Read the model definition and answer for the solid it produces. Units are mm, in the model's axes. Face numbers are marked on the shaded views. A direction names the side the tool comes from. Give positions to 0.01 mm unless a question says otherwise; leave off trailing zeros. Loops run counter-clockwise (first coordinate to the right, second up) from the corner with the lowest first, then second, coordinate; pieces in that order, holes last. Notation, with made-up numbers: (43, 37.25) - (47, 37.25) arc R17 cw to (47, 42.25) - close; hole circle Ø6 at (-11, 55.25). An arc over 180 degrees is marked (long way). Write item = value, one per line.
```python
from build123d import *

# Parameters (mm, degrees)
ESBO_O1_W                = 8.5
ESBO_O1_H                = 8.5
ESBO_O1_W_2              = 3.29
ESBO_O1_H_2              = 3.29
RESSALTO_EXTRUS_O1_DEPTH = 7.3
ESBO_O2_W                = 40
ESBO_O2_H                = 40
RESSALTO_EXTRUS_O2_DEPTH = 10
FILETE1_R                = 10
FILETE2_R                = 10
FILETE3_R                = 5
ESBO_O3_W                = 0.5
ESBO_O3_H                = 1.5
ESBO_O3_W_2              = 1.5
ESBO_O3_H_2              = 0.5
CORTE_EXTRUS_O1_DEPTH    = 5
FILETE4_R                = 1


with BuildPart() as part:
    # Esboço1 → Ressalto-extrusão1 (new body)
    with BuildSketch(Plane.XY):
        Rectangle(ESBO_O1_W, ESBO_O1_H)
        Rectangle(ESBO_O1_W_2, ESBO_O1_H_2, mode=Mode.SUBTRACT)
    extrude(amount=RESSALTO_EXTRUS_O1_DEPTH)

    # Esboço2 → Ressalto-extrusão2 (add)
    with BuildSketch(Plane.XY.offset(7.3)):
        Rectangle(ESBO_O2_W, ESBO_O2_H)
    extrude(amount=RESSALTO_EXTRUS_O2_DEPTH)

    # Filete1
    # the kernel refuses this fillet: 10 mm, written as the material it adds along each edge
    with BuildSketch(Plane(origin=(-4.25, -4.25, 7.3), x_dir=(-1, 0, 0), z_dir=(0, 1, 0)), Plane(origin=(4.25, -4.25, 7.3), x_dir=(0, -1, 0), z_dir=(-1, 0, 0)), Plane(origin=(4.25, 4.25, 7.3), x_dir=(1, 0, 0), z_dir=(0, -1, 0)), Plane(origin=(-4.25, 4.25, 7.3), x_dir=(0, 1, 0), z_dir=(1, 0, 0))) as filete1_piece_1:
        with BuildLine():
            CenterArc((9.628603222, -10), FILETE1_R, 90, 74.335733149)
            Line((0, -7.3), (-0.192572064, -7.246))
            ThreePointArc((-0.192572064, -7.246), (-0.2, -3.65), (-0.2, 0))
            Line((-0.2, 0), (0, 0.2))
            Line((0, 0.2), (9.628603222, 0.2))
            Line((9.628603222, 0.2), (9.628603222, 0))
        make_face()
    extrude(amount=8.5)
    with BuildSketch(Plane(origin=(4.25, -4.25, 7.3), x_dir=(0, -1, 0), z_dir=(-1, 0, 0))) as filete1_piece_2a_section:
        with BuildLine():
            CenterArc((9.628603222, -10), FILETE1_R, 90, 74.335733149)
            Line((0, -7.3), (-0.192572064, -7.246))
            ThreePointArc((-0.192572064, -7.246), (-0.2, -3.65), (-0.2, 0))
            Line((-0.2, 0), (0, 0.2))
            Line((0, 0.2), (9.628603222, 0.2))
            Line((9.628603222, 0.2), (9.628603222, 0))
        make_face()
    filete1_piece_2a = extrude(amount=32.571508054, mode=Mode.PRIVATE)
    filete1_piece_2a = split(filete1_piece_2a, bisect_by=Plane(origin=(-20, -6.528048656, 5.446397175), z_dir=(1, 0, 0)), keep=Keep.TOP, mode=Mode.PRIVATE)
    filete1_piece_2a = split(filete1_piece_2a, bisect_by=Plane(origin=(-4.25, -6.528048656, 5.446397175), z_dir=(-1, 0, 0)), keep=Keep.TOP, mode=Mode.PRIVATE)
    with BuildSketch(Plane(origin=(-4.25, -28.321508054, 7.3), x_dir=(-1, 0, 0), z_dir=(0, 1, 0))) as filete1_piece_2b_section:
        with BuildLine():
            CenterArc((9.628603222, -10), FILETE1_R, 90, 74.335733149)
            Line((0, -7.3), (-0.192572064, -7.246))
            ThreePointArc((-0.192572064, -7.246), (-0.2, -3.65), (-0.2, 0))
            Line((-0.2, 0), (0, 0.2))
            Line((0, 0.2), (9.628603222, 0.2))
            Line((9.628603222, 0.2), (9.628603222, 0))
        make_face()
    filete1_piece_2b = extrude(amount=32.571508054, mode=Mode.PRIVATE)
    filete1_piece_2b = split(filete1_piece_2b, bisect_by=Plane(origin=(-6.528048656, -20, 5.446397175), z_dir=(0, 1, 0)), keep=Keep.TOP, mode=Mode.PRIVATE)
    filete1_piece_2b = split(filete1_piece_2b, bisect_by=Plane(origin=(-6.528048656, -4.25, 5.446397175), z_dir=(0, -1, 0)), keep=Keep.TOP, mode=Mode.PRIVATE)
    filete1_piece_2 = filete1_piece_2a & filete1_piece_2b
    add(filete1_piece_2)
    with BuildSketch(Plane(origin=(-28.321508054, 4.25, 7.3), x_dir=(0, 1, 0), z_dir=(1, 0, 0))) as filete1_piece_3a_section:
        with BuildLine():
            CenterArc((9.628603222, -10), FILETE1_R, 90, 74.335733149)
            Line((0, -7.3), (-0.192572064, -7.246))
            ThreePointArc((-0.192572064, -7.246), (-0.2, -3.65), (-0.2, 0))
            Line((-0.2, 0), (0, 0.2))
            Line((0, 0.2), (9.628603222, 0.2))
            Line((9.628603222, 0.2), (9.628603222, 0))
        make_face()
    filete1_piece_3a = extrude(amount=32.571508054, mode=Mode.PRIVATE)
    filete1_piece_3a = split(filete1_piece_3a, bisect_by=Plane(origin=(-20, 6.528048656, 5.446397175), z_dir=(1, 0, 0)), keep=Keep.TOP, mode=Mode.PRIVATE)
    filete1_piece_3a = split(filete1_piece_3a, bisect_by=Plane(origin=(-4.25, 6.528048656, 5.446397175), z_dir=(-1, 0, 0)), keep=Keep.TOP, mode=Mode.PRIVATE)
    with BuildSketch(Plane(origin=(-4.25, -4.25, 7.3), x_dir=(-1, 0, 0), z_dir=(0, 1, 0))) as filete1_piece_3b_section:
        with BuildLine():
            CenterArc((9.628603222, -10), FILETE1_R, 90, 74.335733149)
            Line((0, -7.3), (-0.192572064, -7.246))
            ThreePointArc((-0.192572064, -7.246), (-0.2, -3.65), (-0.2, 0))
            Line((-0.2, 0), (0, 0.2))
            Line((0, 0.2), (9.628603222, 0.2))
            Line((9.628603222, 0.2), (9.628603222, 0))
        make_face()
    filete1_piece_3b = extrude(amount=32.571508054, mode=Mode.PRIVATE)
    filete1_piece_3b = split(filete1_piece_3b, bisect_by=Plane(origin=(-6.528048656, 20, 5.446397175), z_dir=(0, -1, 0)), keep=Keep.TOP, mode=Mode.PRIVATE)
    filete1_piece_3b = split(filete1_piece_3b, bisect_by=Plane(origin=(-6.528048656, 4.25, 5.446397175), z_dir=(0, 1, 0)), keep=Keep.TOP, mode=Mode.PRIVATE)
    filete1_piece_3 = filete1_piece_3a & filete1_piece_3b
    add(filete1_piece_3)
    with BuildSketch(Plane(origin=(4.25, 4.25, 7.3), x_dir=(1, 0, 0), z_dir=(0, -1, 0))) as filete1_piece_4a_section:
        with BuildLine():
            CenterArc((9.628603222, -10), FILETE1_R, 90, 74.335733149)
            Line((0, -7.3), (-0.192572064, -7.246))
            ThreePointArc((-0.192572064, -7.246), (-0.2, -3.65), (-0.2, 0))
            Line((-0.2, 0), (0, 0.2))
            Line((0, 0.2), (9.628603222, 0.2))
            Line((9.628603222, 0.2), (9.628603222, 0))
        make_face()
    filete1_piece_4a = extrude(amount=32.571508054, mode=Mode.PRIVATE)
    filete1_piece_4a = split(filete1_piece_4a, bisect_by=Plane(origin=(6.528048656, -20, 5.446397175), z_dir=(0, 1, 0)), keep=Keep.TOP, mode=Mode.PRIVATE)
    filete1_piece_4a = split(filete1_piece_4a, bisect_by=Plane(origin=(6.528048656, -4.25, 5.446397175), z_dir=(0, -1, 0)), keep=Keep.TOP, mode=Mode.PRIVATE)
    with BuildSketch(Plane(origin=(28.321508054, -4.25, 7.3), x_dir=(0, -1, 0), z_dir=(-1, 0, 0))) as filete1_piece_4b_section:
        with BuildLine():
            CenterArc((9.628603222, -10), FILETE1_R, 90, 74.335733149)
            Line((0, -7.3), (-0.192572064, -7.246))
            ThreePointArc((-0.192572064, -7.246), (-0.2, -3.65), (-0.2, 0))
            Line((-0.2, 0), (0, 0.2))
            Line((0, 0.2), (9.628603222, 0.2))
            Line((9.628603222, 0.2), (9.628603222, 0))
        make_face()
    filete1_piece_4b = extrude(amount=32.571508054, mode=Mode.PRIVATE)
    filete1_piece_4b = split(filete1_piece_4b, bisect_by=Plane(origin=(20, -6.528048656, 5.446397175), z_dir=(-1, 0, 0)), keep=Keep.TOP, mode=Mode.PRIVATE)
    filete1_piece_4b = split(filete1_piece_4b, bisect_by=Plane(origin=(4.25, -6.528048656, 5.446397175), z_dir=(1, 0, 0)), keep=Keep.TOP, mode=Mode.PRIVATE)
    filete1_piece_4 = filete1_piece_4a & filete1_piece_4b
    add(filete1_piece_4)
    with BuildSketch(Plane(origin=(-4.25, 4.25, 7.3), x_dir=(0, 1, 0), z_dir=(1, 0, 0))) as filete1_piece_5a_section:
        with BuildLine():
            CenterArc((9.628603222, -10), FILETE1_R, 90, 74.335733149)
            Line((0, -7.3), (-0.192572064, -7.246))
            ThreePointArc((-0.192572064, -7.246), (-0.2, -3.65), (-0.2, 0))
            Line((-0.2, 0), (0, 0.2))
            Line((0, 0.2), (9.628603222, 0.2))
            Line((9.628603222, 0.2), (9.628603222, 0))
        make_face()
    filete1_piece_5a = extrude(amount=32.571508054, mode=Mode.PRIVATE)
    filete1_piece_5a = split(filete1_piece_5a, bisect_by=Plane(origin=(20, 6.528048656, 5.446397175), z_dir=(-1, 0, 0)), keep=Keep.TOP, mode=Mode.PRIVATE)
    filete1_piece_5a = split(filete1_piece_5a, bisect_by=Plane(origin=(4.25, 6.528048656, 5.446397175), z_dir=(1, 0, 0)), keep=Keep.TOP, mode=Mode.PRIVATE)
    with BuildSketch(Plane(origin=(4.25, 28.321508054, 7.3), x_dir=(1, 0, 0), z_dir=(0, -1, 0))) as filete1_piece_5b_section:
        with BuildLine():
            CenterArc((9.628603222, -10), FILETE1_R, 90, 74.335733149)
            Line((0, -7.3), (-0.192572064, -7.246))
            ThreePointArc((-0.192572064, -7.246), (-0.2, -3.65), (-0.2, 0))
            Line((-0.2, 0), (0, 0.2))
            Line((0, 0.2), (9.628603222, 0.2))
            Line((9.628603222, 0.2), (9.628603222, 0))
        make_face()
    filete1_piece_5b = extrude(amount=32.571508054, mode=Mode.PRIVATE)
    filete1_piece_5b = split(filete1_piece_5b, bisect_by=Plane(origin=(6.528048656, 20, 5.446397175), z_dir=(0, -1, 0)), keep=Keep.TOP, mode=Mode.PRIVATE)
    filete1_piece_5b = split(filete1_piece_5b, bisect_by=Plane(origin=(6.528048656, 4.25, 5.446397175), z_dir=(0, 1, 0)), keep=Keep.TOP, mode=Mode.PRIVATE)
    filete1_piece_5 = filete1_piece_5a & filete1_piece_5b
    add(filete1_piece_5)

    # Filete2
    filete2_edges = [part.edges().sort_by_distance(p)[0] for p in [
        (-20, 20, 12.3),
        (-20, -20, 12.3),
        (20, -20, 12.3),
        (20, 20, 12.3),
    ]]
    fillet(filete2_edges, radius=FILETE2_R)

    # Filete3
    filete3_edges = [part.edges().sort_by_distance(p)[0] for p in [
        (0, 20, 17.3),
        (20, 0, 17.3),
        (-20, 0, 17.3),
        (0, -20, 17.3),
        (-17.071067812, 17.071067812, 17.3),
        (-17.071067812, -17.071067812, 17.3),
        (17.071067812, -17.071067812, 17.3),
        (17.071067812, 17.071067812, 17.3),
    ]]
    fillet(filete3_edges, radius=FILETE3_R)

    # Esboço3 → Corte-extrusão1 (cut)
    with BuildSketch(Plane(origin=(0, 0, 0), x_dir=(-1, 0, 0), z_dir=(0, 0, -1))):
        with Locations((0, 2.395)):
            Rectangle(ESBO_O3_W, ESBO_O3_H)
        with Locations((0, -2.395)):
            Rectangle(ESBO_O3_W, ESBO_O3_H)
        with Locations((2.395, 0)):
            Rectangle(ESBO_O3_W_2, ESBO_O3_H_2)
        with Locations((-2.395, 0)):
            Rectangle(ESBO_O3_W_2, ESBO_O3_H_2)
    extrude(amount=-CORTE_EXTRUS_O1_DEPTH, mode=Mode.SUBTRACT)

    # Filete4
    filete4_edges = [part.edges().sort_by_distance(p)[0] for p in [
        (0, 20, 7.3),
        (-20, 0, 7.3),
        (20, 0, 7.3),
        (0, -20, 7.3),
        (-17.071067812, 17.071067812, 7.3),
        (-17.071067812, -17.071067812, 7.3),
        (17.071067812, -17.071067812, 7.3),
        (17.071067812, 17.071067812, 7.3),
    ]]
    fillet(filete4_edges, radius=FILETE4_R)


solid = part.part
```
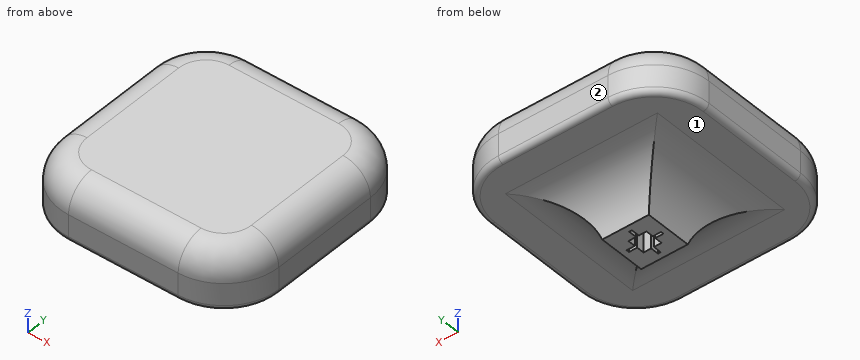
1) Each of these flat-tipped pins is pushed along its axis until it touches: P1, Ø1.6, axis at y = -0.5, z = 4, coming from the -X side; P2, Ø1.6, axis at x = 2.5, z = 3, coming from the +Y side; P3, Ø1, axis at x = -7.5, y = -5, coming from the -Z side; P4, Ø2, axis at x = 9, z = 3.5, coming from the +Y side. Where does it stop, or does it pass through?
Output:
P1 = -7.26
P2 = 6.28
P3 = 4.56
P4 = through
2) A cutting plane is placed at A-A on z = 2.75. Determine the outline of the cut face in (x, y) (3 decimals).
Output:
outline = (-5.494, -5.494) - (5.494, -5.494) - (5.494, 5.494) - (-5.494, 5.494) - close; hole (-3.145, -0.25) - (-1.645, -0.25) - (-1.645, -1.645) - (-0.25, -1.645) - (-0.25, -3.145) - (0.25, -3.145) - (0.25, -1.645) - (1.645, -1.645) - (1.645, -0.25) - (3.145, -0.25) - (3.145, 0.25) - (1.645, 0.25) - (1.645, 1.645) - (0.25, 1.645) - (0.25, 3.145) - (-0.25, 3.145) - (-0.25, 1.645) - (-1.645, 1.645) - (-1.645, 0.25) - (-3.145, 0.25) - close
3) Find the intervals of material crossed by probe 1 along X at (y, z) = (0.5, 3) (3 decimals); probe 2 along Z at (x, y) = (-15, -8.5); probe 3 along X at (y, z) = (-3, 3), in increasing order.
Output:
probe_1 = -5.662 to -1.645, 1.645 to 5.662
probe_2 = 7.3 to 17.3
probe_3 = -5.66 to -0.25, 0.25 to 5.66
4) A tool of negligible diameter and unlimited length cuts with its end or side. For the marked faces 1 and 2, from which of +Z, -Z, +X, -X, +Y, -Y can it reach the whole face along a straight path? Write none if from no direction.
Output:
face_1 = -Z
face_2 = +Z, -Z, +X, -X, +Y
5) A cutting plane is placed at C-C on z = 9.75. Determine the outline of the cut face in (x, y).
Output:
outline = (-20, -10) arc R10 ccw to (-10, -20) - (10, -20) arc R10 ccw to (20, -10) - (20, 10) arc R10 ccw to (10, 20) - (-10, 20) arc R10 ccw to (-20, 10) - close
6) A cutting plane is placed at B-B on y = 6. Determine the outline of the cut face in (x, z), then the cut area to 3 significant figures.
Output:
outline = (-20, 8.3) arc R1 ccw to (-19, 7.3) - (-13.88, 7.3) arc R10 cw to (-6, 3.46) - (6, 3.46) arc R10 cw to (13.88, 7.3) - (19, 7.3) arc R1 ccw to (20, 8.3) - (20, 12.3) arc R5 ccw to (15, 17.3) - (-15, 17.3) arc R5 ccw to (-20, 12.3) - close
area = 453 mm²
